```python
from build123d import *

# Parameters (mm, degrees)
SKETCH2_R           = 23
SKETCH2_R_2         = 20.625
BOSS_EXTRUDE1_DEPTH = 10
SKETCH3_W           = 2.53
SKETCH3_H           = 8.74
BOSS_EXTRUDE2_DEPTH = 10
CIRPATTERN1_COUNT   = 6
SKETCH4_W           = 1.15
SKETCH4_H           = 2.3


with BuildPart() as part:
    # Sketch2 → Boss-Extrude1 (new body)
    with BuildSketch(Plane.XY):
        Circle(SKETCH2_R)
        Circle(SKETCH2_R_2, mode=Mode.SUBTRACT)
    extrude(amount=BOSS_EXTRUDE1_DEPTH)

    # Sketch3 → Boss-Extrude2 (add)
    with BuildSketch(Plane.XY):
        with Locations((-19.5, 0)):
            Rectangle(SKETCH3_W, SKETCH3_H)
    boss_extrude2 = extrude(amount=BOSS_EXTRUDE2_DEPTH)

    # CirPattern1: Boss-Extrude2 ×6 about axis
    cirpattern1_axis = Axis((0, 0, 0), (0, 0, 1))
    for i in range(1, CIRPATTERN1_COUNT):
        add(boss_extrude2.rotate(cirpattern1_axis, i * 360 / CIRPATTERN1_COUNT))

    # Sketch4 → Cut-Revolve1 (revolve, cut)
    with BuildSketch(Plane(origin=(0, 0, 0), x_dir=(0, 0, -1), z_dir=(1, 0, 0))):
        with Locations((-5, 23)):
            Rectangle(SKETCH4_W, SKETCH4_H)
    revolve(axis=Axis((0, 0, 10), (0, 0, -1)), mode=Mode.SUBTRACT)


solid = part.part
```
Can you work these out from the model? Positions are in its coordinate system, mm. A direction names the side the tool comes from. Give positions to 0.01 mm unless a question says otherwise; leave off trailing zeros. Order: outer loops, then holes, each group sorted by start corner. A loop starts at its lowest first (then second) coordinate and runs counter-clockwise, first axis right, second up. Notation, with made-up numbers: M -30.75,7 L -2.75,7 A14 ccw -2.75,14 Z; hole C -40,-20.75 d11. An arc over 180 degrees is marked long. Write item = value, one per line. Start each with the question number.
Q1. Suppose I cut it at B-B (x = 0). Write out the boundary of the cut face in (y, z) (3 decimals), plus the area to 3 significant figures.
Q2. Suppose I cut it at D-D (z = 5). Write out the boundary of the cut face in (x, y) (3 decimals), plus the area to 3 significant figures.
Q3. Suppose I cut it at A-A (y = 0). Write out the boundary of the cut face in (x, z) (3 decimals), plus the area to 3 significant figures.
Q4. I need wall thicknesses on probe 1 along X at (y, z) = (0, 1) (3 decimals); probe 2 along Z at (x, y) = (20.5, -8) (3 decimals); probe 3 along X at (y, z) = (9, 1.5). Which ranges of each line are inside material? Lowest first, please. Write a range as [from, to].
Q5. Will these pins go through, and if not, where does the flat tip stop? pin 1 Ø3 at (x, y) = (3, -18) entering from +Z; pin 2 Ø3 at (x, z) = (-4.5, 5) entering from +Y; pin 3 Ø1 at (y, z) = (-5.5, 5.5) entering from +X; pin 4 Ø23 at (x, y) = (-4.5, -5.5) entering from +Z.
Q6. We'd pull the mould along Y, two halves only. Please class faces 1 (the flat face through (18.235, 0, 5)), 2 (the cylindrical face through (-2.994, 22.804, 2.182)), 3 (the flat face through (11, 15, 10)): pulls with the +Y half, pulls with the -Y half, needs draft (parallel to the pull), parting line crosses it, or undercut.
Q7. Suppose I cut it at C-C (z = 2.5). Write out the boundary of the cut face in (x, y) (3 decimals), plus the area to 3 significant figures.
Q8. For faces 4 (the flat face through (-8.41, -20.34, 4.425)), 5 (the flat face through (-19, -4.37, 5)), 6 (the flat face through (-10.3, 15.4, 0)), which set-ups out of +Z, -Z, +X, -X, +Y, -Y let a thin tool reach every point of the face, with its end or its side?
Check result:
q1.outline = M -23,0 L -20.625,0 L -20.625,10 L -23,10 L -23,5.575 L -21.85,5.575 L -21.85,4.425 L -23,4.425 Z; M 20.625,0 L 23,0 L 23,4.425 L 21.85,4.425 L 21.85,5.575 L 23,5.575 L 23,10 L 20.625,10 Z
q1.area = 44.9 mm2
q2.outline = C 0,0 d43.7; hole M -20.157,-4.37 A20.625 ccw -13.863,-15.271 L -12.902,-13.607 L -5.333,-17.977 L -6.294,-19.641 A20.625 ccw 6.294,-19.641 L 5.333,-17.977 L 12.902,-13.607 L 13.863,-15.271 A20.625 ccw 20.157,-4.37 L 18.235,-4.37 L 18.235,4.37 L 20.157,4.37 A20.625 ccw 13.863,15.271 L 12.902,13.607 L 5.333,17.977 L 6.294,19.641 A20.625 ccw -6.294,19.641 L -5.333,17.977 L -12.902,13.607 L -13.863,15.271 A20.625 ccw -20.157,4.37 L -18.235,4.37 L -18.235,-4.37 Z
q2.area = 281 mm2
q3.outline = M -23,0 L -18.235,0 L -18.235,10 L -23,10 L -23,5.575 L -21.85,5.575 L -21.85,4.425 L -23,4.425 Z; M 18.235,0 L 23,0 L 23,4.425 L 21.85,4.425 L 21.85,5.575 L 23,5.575 L 23,10 L 18.235,10 Z
q3.area = 92.7 mm2
q4.probe_1 = [-23, -18.235], [18.235, 23]
q4.probe_2 = [0, 4.425], [5.575, 10]
q4.probe_3 = [-21.17, -18.56], [18.56, 21.17]
q5.pin_1 = through
q5.pin_2 = 22.79
q5.pin_3 = 22.45
q5.pin_4 = 10
q6.face_1 = undercut
q6.face_2 = parting line crosses it
q6.face_3 = needs draft
q7.outline = C 0,0 d46; hole M -20.157,-4.37 A20.625 ccw -13.863,-15.271 L -12.902,-13.607 L -5.333,-17.977 L -6.294,-19.641 A20.625 ccw 6.294,-19.641 L 5.333,-17.977 L 12.902,-13.607 L 13.863,-15.271 A20.625 ccw 20.157,-4.37 L 18.235,-4.37 L 18.235,4.37 L 20.157,4.37 A20.625 ccw 13.863,15.271 L 12.902,13.607 L 5.333,17.977 L 6.294,19.641 A20.625 ccw -6.294,19.641 L -5.333,17.977 L -12.902,13.607 L -13.863,15.271 A20.625 ccw -20.157,4.37 L -18.235,4.37 L -18.235,-4.37 Z
q7.area = 443 mm2
q8.face_4 = none
q8.face_5 = +Z, -Z
q8.face_6 = -Z, +X, -X, +Y, -Y
